Check sheet for the drawn part. Datum: minimum x, y, z corner. Units: mm. Coordinates: 2 decimals unless noted, no trailing zeros. Write each loop counter-clockwise with the first axis right and the second up, starting at its lowest first coordinate (ties: lowest second). Pieces come first, ordered by that corner, then holes. Notation, with made-up numbers: (-40, 0.5) -> (0, 0.5) arc R29 ccw to (0, 23.5) -> close; hole circle Ø5 at (-35.5, 77.25). An arc over 180 degrees is marked (long way). Answer in a Markdown table with one row per item. Add a question column.
1. Cross-section at B-B on x = 9. Record the cut outline in (y, z), and give its area (3 significant figures).
2. Cross-section at A-A on y = 10. Record the cut outline in (x, z), and give its area (3 significant figures).
3. Mould release check, pull along Y, two halves, no side actions. Record for the marked faces 1, 2, 3 and 4: pulls with the +Y half, pulls with the -Y half, needs draft (parallel to the pull), parting line crosses it, or undercut.
4. Cross-section at C-C on z = 2.75. Record the cut outline in (x, y), and give its area (3 significant figures).
5. Cross-section at D-D on y = 28. Record the cut outline in (x, z).
6. Scan lines: L1, parallel to Y at x = 9, z = 2.7; L2, parallel to Y at x = 6.75, z = 1.5; L3, parallel to X at y = 28, z = 0.95. Record each from-to range of solid material in increasing order. Write a range as from..to.
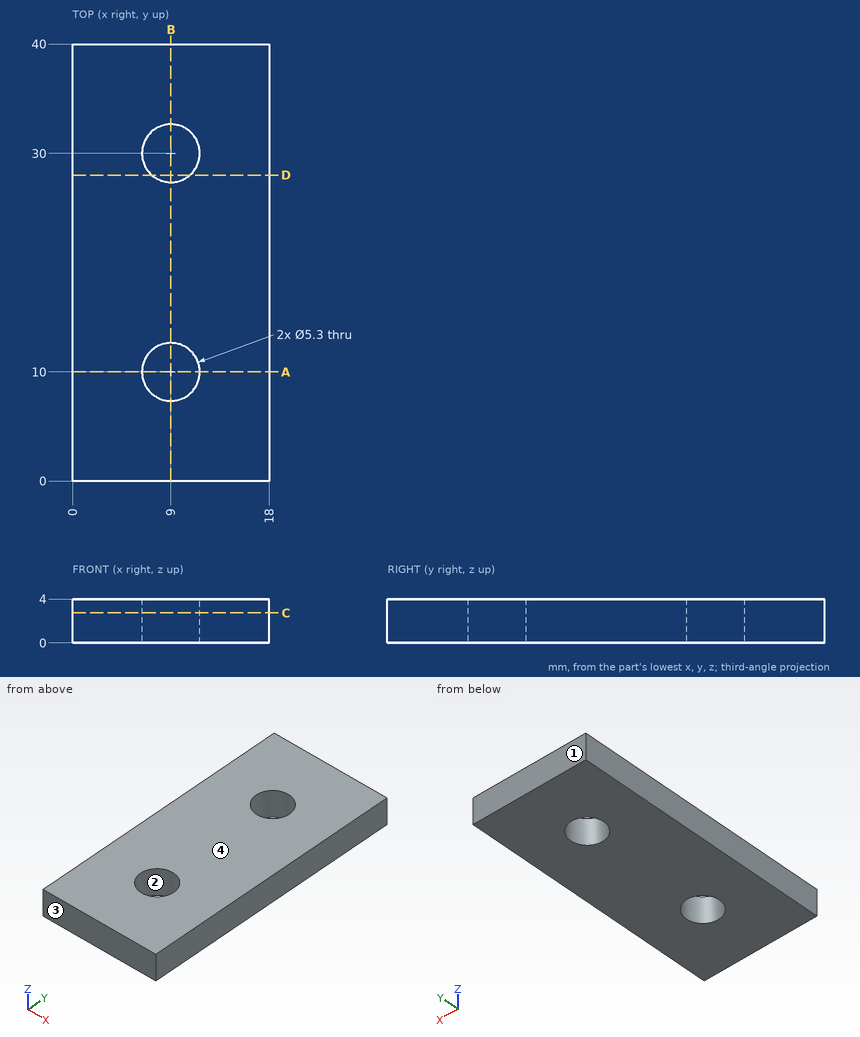
Results found:
| question | item | result |
|---|---|---|
| 1 | outline | (0, 0) -> (7.35, 0) -> (7.35, 4) -> (0, 4) -> close; (12.65, 0) -> (27.35, 0) -> (27.35, 4) -> (12.65, 4) -> close; (32.65, 0) -> (40, 0) -> (40, 4) -> (32.65, 4) -> close |
| 1 | area | 118 mm^2 |
| 2 | outline | (0, 0) -> (6.35, 0) -> (6.35, 4) -> (0, 4) -> close; (11.65, 0) -> (18, 0) -> (18, 4) -> (11.65, 4) -> close |
| 2 | area | 50.8 mm^2 |
| 3 | face 1 | pulls with the +Y half |
| 3 | face 2 | undercut |
| 3 | face 3 | pulls with the -Y half |
| 3 | face 4 | needs draft |
| 4 | outline | (0, 0) -> (18, 0) -> (18, 40) -> (0, 40) -> close; hole circle Ø5.3 at (9, 10); hole circle Ø5.3 at (9, 30) |
| 4 | area | 676 mm^2 |
| 5 | outline | (0, 0) -> (7.26, 0) -> (7.26, 4) -> (0, 4) -> close; (10.74, 0) -> (18, 0) -> (18, 4) -> (10.74, 4) -> close |
| 6 | L1 | y = 0..7.35, 12.65..27.35, 32.65..40 |
| 6 | L2 | y = 0..8.6, 11.4..28.6, 31.4..40 |
| 6 | L3 | x = 0..7.26, 10.74..18 |
